CAD build for the part. Positions are in the model's coordinates, mm. A direction names the side the tool comes from. Round coordinates to 2 decimals unless told otherwise and drop trailing zeros. Write each loop counter-clockwise with the first axis right and the second up, starting at its lowest first coordinate (ties: lowest second). Pieces come first, ordered by that corner, then holes. Notation, with made-up numbers: (34.5, 34.25) -> (45.5, 34.25) arc R18 ccw to (45.5, 54.25) -> close; hole circle Ø7 at (34, 3.5). An arc over 180 degrees is marked (long way). Put each result on its own line as item: value. Start each with the question number.
1. Saw through at A-A on y = -11. List the corners of the cut face in (x, z), and give its area (3 significant figures).
2. Drill centre lines: line 1 (Y direction, x = 16.5, z = 5); line 2 (Z direction, x = -9, y = -30); line 3 (Z direction, x = -12, y = 30.5). Where is each one in solid material? Low to high. Write a range as from..to.
3. Flat gauge pins, fed straight in: P1, Ø6, axis at y = 8.5, z = 22.5, coming from the -X side; P2, Ø1.8, axis at y = -12, z = 4, coming from the -X side; P3, Ø1.5, axis at x = -38, z = 15.5, coming from the -Y side. Where does each tip first touch, or does it go through?
4. 3-axis set-ups, long thin cutter, end or side, ignore diameter. For faces 1 (the flat face through (23, -26.1, 4)), 2 (the flat face through (-46, 29, 35)), 3 (the flat face through (28, 0, 6)), 4 (the flat face through (-38.1, 0.5, 0.3)), 5 (the flat face through (-11, 26.1, 3)): which of +Z, -Z, +X, -X, +Y, -Y reach the whole face in a straight line?
5. Saw through at B-B on x = -15. State how many separate pieces and enclosed holes the cut face has, and give its area (3 significant figures).
6. Pull direction Y, two halves, no side cores. Call faces 6 (the flat face through (-45, -29, 35)), 7 (the flat face through (26.1, 0, 3)), 8 (the flat face through (-45.58, 0.2, 16.54)): pulls with the +Y half, pulls with the -Y half, needs draft (parallel to the pull), parting line crosses it, or undercut.
from build123d import *

# Parameters (mm, degrees)
F0_W        = 12
F0_H        = 12
F0_H_2      = 28
F1_DEPTH    = 6
F3_W        = 28
F3_H        = 35
F4_DEPTH    = 13.2
F6_W        = 11.9632627889
F6_H        = 28
F9_DEPTH    = 15
F11_DEPTH   = 15
F12_DEPTH   = 0.42144
F9_FACE_W   = 14.5645885303
F9_FACE_H   = 15
F11_FACE1_W = 14.5645885303
F11_FACE1_H = 15


with BuildPart() as f1:
    # F0 (on Top) → F1 (new body)
    with BuildSketch(Plane.XY):
        Polygon((38.1, -38.1), (38.1, 38.1), (26.1, 38.1), (26.1, 26.1), (26.1, -26.1), (26.1, -38.1), align=None)
        with Locations((20.1, 32.1)):
            Rectangle(F0_W, F0_H)
        Polygon((14.1, 26.1), (14.1, 38.1), (-13.07, 38.1), (-26.1, 38.1), (-26.1, 26.1), (-12.9487672821, 26.1), align=None)
        with Locations((20.1, -32.1)):
            Rectangle(F0_W, F0_H)
        Polygon((-13.07, -38.1), (14.1, -38.1), (14.1, -26.1), (-12.9487672821, -26.1), (-26.1, -26.1), (-26.1, -38.1), align=None)
        Polygon((-26.1, 26.1), (-26.1, 38.1), (-38.1, 38.1), (-38.1, 14), (-26.1, 14), align=None)
        Polygon((-38.1, -38.1), (-26.1, -38.1), (-26.1, -26.1), (-26.1, -14), (-38.1, -14), (-38.1, -20), (-38.1, -23), align=None)
        with Locations((-32.1, 0)):
            Rectangle(F0_W, F0_H_2)
    extrude(amount=F1_DEPTH)

    # F3 (on face) → F4 (join)
    with BuildSketch(Plane(origin=(-19.1402449771, 0, -8.9252428118), x_dir=(0, -1, 0), z_dir=(-0.906307787, 0, -0.4226182617))):
        with Locations((0, 33.9681833537)):
            Rectangle(F3_W, F3_H)
    extrude(amount=F4_DEPTH)

    # F6 (on face) → F7 (join, up to the next surface of F1)
    with BuildSketch(Plane.XY.offset(37.7207725463)):
        with Locations((-46.8732705554, 0)):
            Rectangle(F6_W, F6_H)
    extrude(until=Until.NEXT, dir=(0, 0, -1))

    # F8 (on face) → F9 (join)
    with BuildSketch(Plane(origin=(0, 14, 0), x_dir=(-1, 0, 0), z_dir=(0, 1, 0))):
        Polygon((38.2903134195, 32.1422114913), (52.8549019498, 32.1422114913), (52.8549019498, 37.7207725463), (40.8916391609, 37.7207725463), align=None)
    extrude(amount=F9_DEPTH)

    # F10 (on face) → F11 (join)
    with BuildSketch(Plane.XZ.offset(14)):
        Polygon((-52.8549019498, 37.7207725463), (-52.8549019498, 32.1422114913), (-38.2903134195, 32.1422114913), (-40.8916391609, 37.7207725463), align=None)
    extrude(amount=F11_DEPTH)

    # F12 (add): a face of the model
    f12_faces = [f1.faces().sort_by_distance(p)[0] for p in [
        (-46.8732705554, 0, 37.7207725463),
    ]]
    extrude(f12_faces, amount=F12_DEPTH)

    # F9_face (on face) → F13 section 0
    with BuildSketch(Plane(origin=(-45.5726076847, 21.5, 32.1422114913), x_dir=(1, 0, 0), z_dir=(0, 0, -1))):
        Rectangle(F9_FACE_W, F9_FACE_H)
    # F0 (on Top) → F13 section 1
    with BuildSketch(Plane.XY):
        with Locations((20.1, 32.1)):
            Rectangle(F0_W, F0_H)
    loft()

    # F11_face1 (on face) → F14 section 0
    with BuildSketch(Plane(origin=(-45.5726076847, -21.5, 32.1422114913), x_dir=(1, 0, 0), z_dir=(0, 0, -1))):
        Rectangle(F11_FACE1_W, F11_FACE1_H)
    # F0 (on Top) → F14 section 1
    with BuildSketch(Plane.XY):
        with Locations((20.1, -32.1)):
            Rectangle(F0_W, F0_H)
    loft()


solid = f1.part
Return value:
1. outline: (-52.85, 32.14) -> (-38.1, 0.5) -> (-38.1, 0) -> (-26.1, 0) -> (-26.1, 6) -> (-40.89, 37.72) -> (-40.89, 38.14) -> (-52.85, 38.14) -> close; (26.1, 0) -> (38.1, 0) -> (38.1, 6) -> (26.1, 6) -> close
1. area: 611 mm^2
2. line 1: y = -38.1..-26.1, 26.1..38.1
2. line 2: z = 0..6, 11.09..17.52
2. line 3: z = 0..6, 12.53..19.02
3. P1: stops at x = -49.76
3. P2: stops at x = -40.15
3. P3: stops at y = -14
4. face 1: +Z
4. face 2: +Z, +X, -X, +Y
4. face 3: none
4. face 4: -Z, -X
4. face 5: -Z
5. separate pieces: 4
5. enclosed holes: 0
5. area: 322 mm^2
6. face 6: pulls with the -Y half
6. face 7: undercut
6. face 8: needs draft
